The drawing under review shows one solid part. Ordinate dimensions are in mm from its lowest x, y, z. A direction names the side the tool comes from. Coordinates: 2 decimals unless noted, no trailing zeros. Loops run counter-clockwise (first coordinate to the right, second up) from the corner with the lowest first, then second, coordinate; pieces in that order, holes last. Notation, with made-up numbers: (-20.75, 43) -> (-14.75, 43) arc R22 cw to (-14.75, 58) -> close; hole circle Ø10 at (75.25, 42.5). An arc over 180 degrees is marked (long way). Use a Markdown table: item, result.
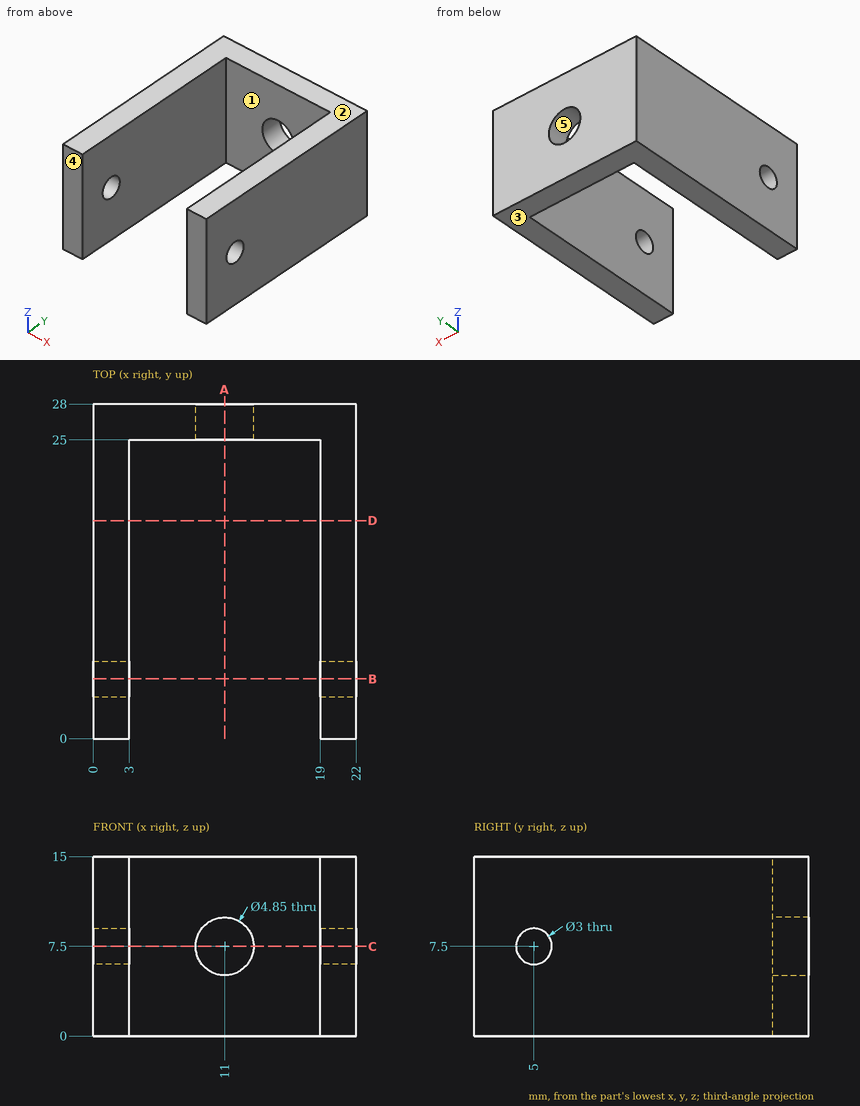
(1) Take a section at A-A on x = 11. Write out the cut boundary in (y, z) (3 decimals).
Found:
| item | result |
|---|---|
| outline | (25, 0) -> (28, 0) -> (28, 5.075) -> (25, 5.075) -> close; (25, 9.925) -> (28, 9.925) -> (28, 15) -> (25, 15) -> close |
(2) For pin 1 Ø4.5 at (x, z) = (13, 7) entering from -Y, flat-tipped, find the tip position at first contact; note if it passes through.
Found:
| item | result |
|---|---|
| pin 1 | stops at y = 25 |
(3) Take a section at B-B on y = 5. Write out the cut boundary in (x, z), plus the area to 3 significant figures.
Found:
| item | result |
|---|---|
| outline | (0, 0) -> (3, 0) -> (3, 6) -> (0, 6) -> close; (0, 9) -> (3, 9) -> (3, 15) -> (0, 15) -> close; (19, 0) -> (22, 0) -> (22, 6) -> (19, 6) -> close; (19, 9) -> (22, 9) -> (22, 15) -> (19, 15) -> close |
| area | 72.0 mm^2 |
(4) For the marked faces 1 and 2, list the 3-axis set-ups (+Z, -Z, +X, -X, +Y, -Y) from which the entire face can be reached by the end or side of a thin tool; tool diameter is ignored.
Found:
| item | result |
|---|---|
| face 1 | +Z, -Z, -Y |
| face 2 | +Z, +X, -X, +Y, -Y |
(5) For line 1 along X through (y, z) = (17.5, 11.25); line 2 along X through (y, z) = (26.45, 7.5) (3 decimals); line 3 along Y through (x, z) = (2.1, 7.5), list the stretches that pass through material, from the lowest coordinate up.
Found:
| item | result |
|---|---|
| line 1 | x = 0 to 3, 19 to 22 |
| line 2 | x = 0 to 8.575, 13.425 to 22 |
| line 3 | y = 0 to 3.5, 6.5 to 28 |
(6) Take a section at C-C on z = 7.5. Write out the cut boundary in (x, y) (3 decimals), plus the area to 3 significant figures.
Found:
| item | result |
|---|---|
| outline | (0, 0) -> (3, 0) -> (3, 3.5) -> (0, 3.5) -> close; (0, 6.5) -> (3, 6.5) -> (3, 25) -> (8.575, 25) -> (8.575, 28) -> (0, 28) -> close; (13.425, 25) -> (19, 25) -> (19, 6.5) -> (22, 6.5) -> (22, 28) -> (13.425, 28) -> close; (19, 0) -> (22, 0) -> (22, 3.5) -> (19, 3.5) -> close |
| area | 183 mm^2 |
(7) Mouldability with a two-part tool opening along Z and no side actions: class the marked faces 3, 4 and 5 as pulls with the +Z half, pulls with the -Z half, needs draft (parallel to the pull), parting line crosses it, or undercut.
Found:
| item | result |
|---|---|
| face 3 | pulls with the -Z half |
| face 4 | needs draft |
| face 5 | undercut |
(8) Take a section at D-D on y = 18.25. Write out the cut boundary in (x, z).
Found:
| item | result |
|---|---|
| outline | (0, 0) -> (3, 0) -> (3, 15) -> (0, 15) -> close; (19, 0) -> (22, 0) -> (22, 15) -> (19, 15) -> close |
